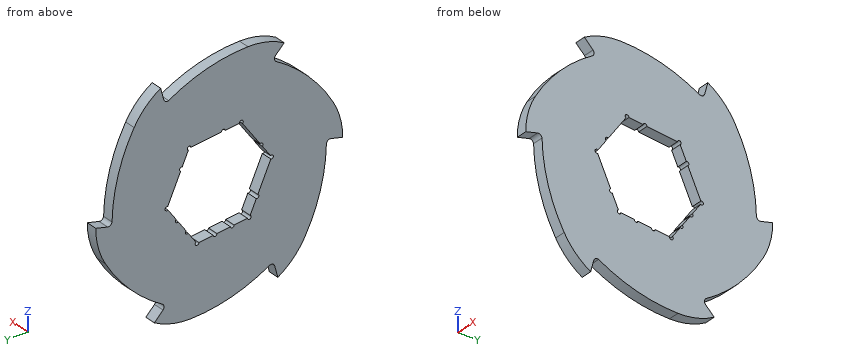
from build123d import *

# Parameters (mm, degrees)
SKETCH1_R                = 59
EXTRUDE1_DEPTH           = 3
EXTRUDE2_DEPTH           = 3
CIRPATTERN1_COUNT        = 6
F_2_0_2_DIAMETER_HOLE1_D = 2
F_2_0_2_DIAMETER_HOLE3_D = 2
F_2_0_2_DIAMETER_HOLE4_D = 2
CIRPATTERN2_COUNT        = 6
CIRPATTERN3_COUNT        = 2
CIRPATTERN3_ANGLE        = 60


with BuildPart() as part:
    # Sketch1 → Extrude1 (new, symmetric)
    with BuildSketch(Plane(origin=(0, 0, 0), x_dir=(0, 0, -1), z_dir=(1, 0, 0))):
        Circle(SKETCH1_R)
        Polygon((26.215177945, 12.224338236), (2.521001516, 28.815179183), (-23.694176429, 16.590840947), (-26.215177945, -12.224338236), (-2.521001516, -28.815179183), (23.694176429, -16.590840947), align=None, mode=Mode.SUBTRACT)
    extrude(amount=EXTRUDE1_DEPTH, both=True)

    # Sketch2 → Extrude2 (add, symmetric)
    with BuildSketch(Plane(origin=(0, 0, 0), x_dir=(0, 0, -1), z_dir=(1, 0, 0))):
        with BuildLine():
            Line((-2, 67.961805723), (-0.262709442, 61.478149092))
            ThreePointArc((-0.262709442, 61.478149092), (-0.58620663, 59.77173183), (-2.122608272, 58.961805723))
            ThreePointArc((-2.122608272, 58.961805723), (28.679663449, 51.560419941), (51.21368579, 29.294340542))
            ThreePointArc((51.21368579, 29.294340542), (36.791707484, 48.186627241), (17.927108603, 62.644803614))
            ThreePointArc((17.927108603, 62.644803614), (8.312130826, 66.609702921), (-2, 67.961805723))
        make_face()
    extrude2 = extrude(amount=EXTRUDE2_DEPTH, both=True)

    # CirPattern1: Extrude2 ×6 about axis
    cirpattern1_axis = Axis((0, 0, 0), (1, 0, 0))
    for i in range(1, CIRPATTERN1_COUNT):
        add(extrude2.rotate(cirpattern1_axis, i * 360 / CIRPATTERN1_COUNT))

    # 2.0 _2_ Diameter Hole1 (through all)
    with Locations(Plane(origin=(3, 0, 0), x_dir=(0, 0, -1), z_dir=(1, 0, 0))):
        with Locations((2.521001516, 28.815179183), (26.215177945, 12.224338236), (23.694176429, -16.590840947), (-2.521001516, -28.815179183), (-26.215177945, -12.224338236), (-23.694176429, 16.590840947)):
            Hole(F_2_0_2_DIAMETER_HOLE1_D / 2)

    # 2.0 _2_ Diameter Hole3 (through all)
    with Locations(Plane(origin=(3, 0, 0), x_dir=(0, 0, -1), z_dir=(1, 0, 0))):
        with Locations((10.692111007, 23.093706722)):
            f_2_0_2_diameter_hole3 = Hole(F_2_0_2_DIAMETER_HOLE3_D / 2)

    # 2.0 _2_ Diameter Hole4 (through all)
    with Locations(Plane(origin=(3, 0, 0), x_dir=(0, 0, -1), z_dir=(1, 0, 0))):
        with Locations((18.453644476, 17.659022479)):
            f_2_0_2_diameter_hole4 = Hole(F_2_0_2_DIAMETER_HOLE4_D / 2)

    # CirPattern2: 2.0 _2_ Diameter Hole3 ×6 about axis
    cirpattern2_axis = Axis((0, 0, 0), (1, 0, 0))
    for i in range(1, CIRPATTERN2_COUNT):
        add(f_2_0_2_diameter_hole3.rotate(cirpattern2_axis, i * 360 / CIRPATTERN2_COUNT), mode=Mode.SUBTRACT)

    # CirPattern3: 2.0 _2_ Diameter Hole4 ×2 about axis
    cirpattern3_axis = Axis((-5.5, 0, 0), (-1, 0, 0))
    for i in range(1, CIRPATTERN3_COUNT):
        add(f_2_0_2_diameter_hole4.rotate(cirpattern3_axis, i * CIRPATTERN3_ANGLE / (CIRPATTERN3_COUNT - 1)), mode=Mode.SUBTRACT)


solid = part.part
Geometry: final body of the model. Coordinates: model frame, mm. Coordinates: 2 decimals unless noted, no trailing zeros. Order: outer loops, then holes, each group sorted by start corner. A loop starts at its lowest first (then second) coordinate and runs counter-clockwise, first axis right, second up.
1) Section C-C (z = 39). Return loops of the section in (x, y).
Result sheet:
outline: (-3, -45.89) - (3, -45.89) - (3, 50.17) - (-3, 50.17) - close
2) Section B-B (y = -26). Return loops of the section in (x, z), then the cut area to 3 significant figures.
Result sheet:
outline: (-3, -53.02) - (3, -53.02) - (3, -3.52) - (-3, -3.52) - close; (-3, 6.54) - (3, 6.54) - (3, 61.87) - (-3, 61.87) - close
area: 629 mm2
3) First-contact query: P1, Ø3, axis at x = -1, y = -7, coming from the -Z side; P2, Ø3, axis at y = -16.59, z = -23.69, coming from the -X side; P3, Ø2, axis at x = 1, z = -40.5, coming from the +Y side; P4, Ø1, axis at x = -1, z = -21, coming from the +Y side. Flat tips, straight axial feed; report the tip coordinate or a pass-through.
Result sheet:
P1: stops at z = -60.71
P2: stops at x = -3
P3: stops at y = 45.35
P4: stops at y = 61.11
4) Ray query, probe 1 along Z at (x, y) = (-1.05, -7); probe 2 along Y at (x, z) = (0.75, 2.5); probe 3 along Z at (x, y) = (-0.9, -12). Return the intervals inside material, ascending.
Result sheet:
probe 1: z = -60.33 to -25.51, 25.76 to 62.8
probe 2: y = -67.71 to -29.81, 26.47 to 58.97
probe 3: z = -58.88 to -24.1, 27.19 to 63.14
5) Section A-A (y = 6.5). Return loops of the section in (x, z), then the cut area to 3 significant figures.
Result sheet:
outline: (-3, -62.75) - (3, -62.75) - (3, -25.71) - (-3, -25.71) - close; (-3, 24.58) - (3, 24.58) - (3, 60.46) - (-3, 60.46) - close
area: 438 mm2
